```python
from build123d import *

# Parameters (mm, degrees)
BASPROSKE_W         = 4.5
BASPROSKE_H         = 48
TOOTHCUT_DEPTH      = 69.031242823
TEETHCUTS_COUNT     = 30
TEETHCUTS_ANGLE     = 348
BORSKE_R            = 5
BORE_DEPTH          = 50.0000508
BOSS_EXTRUDE2_DEPTH = 60
SKETCH6_R           = 7.7
CUT_EXTRUDE2_DEPTH  = 94.547796729


with BuildPart() as part:
    # BasProSke → Base-Revolve (revolve)
    with BuildSketch(Plane(origin=(0, 0, 0), x_dir=(1, 0, 0), z_dir=(0, 1, 0)), mode=Mode.PRIVATE) as base_revolve_sk:
        with Locations((2.25, 24)):
            Rectangle(BASPROSKE_W, BASPROSKE_H)
    revolve(base_revolve_sk.sketch.rotate(Axis((-10, 0, 0), (1, 0, 0)), 180), axis=Axis((-10, 0, 0), (1, 0, 0)))

    # TooCutSke → ToothCut (cut, through all)
    with BuildSketch(Plane(origin=(0, 0, 0), x_dir=(0, 0, -1), z_dir=(1, 0, 0))):
        with BuildLine():
            ThreePointArc((1.388358102, 41.225628713), (0, 41.249), (-1.388358102, 41.225628713))
            ThreePointArc((-1.388358102, 41.225628713), (-2.434419088, 44.674608087), (-4.146627223, 47.846050285))
            ThreePointArc((-4.146627223, 47.846050285), (0, 48.0254), (4.146627223, 47.846050285))
            ThreePointArc((4.146627223, 47.846050285), (2.434419088, 44.674608087), (1.388358102, 41.225628713))
        make_face()
    toothcut = extrude(amount=TOOTHCUT_DEPTH, mode=Mode.SUBTRACT)

    # TeethCuts: ToothCut ×30 about axis
    teethcuts_axis = Axis((-10, 0, 0), (1, 0, 0))
    for i in range(1, TEETHCUTS_COUNT):
        add(toothcut.rotate(teethcuts_axis, i * TEETHCUTS_ANGLE / (TEETHCUTS_COUNT - 1)), mode=Mode.SUBTRACT)

    # BorSke → Bore (cut, symmetric)
    with BuildSketch(Plane(origin=(0, 0, 0), x_dir=(0, 0, -1), z_dir=(1, 0, 0))):
        with Locations(Location((0, 0, 0), (0, 0, 180))):
            Circle(BORSKE_R)
    extrude(amount=BORE_DEPTH, both=True, mode=Mode.SUBTRACT)

    # Sketch5 → Boss-Extrude2 (add)
    with BuildSketch(Plane(origin=(4.5, 0, 0), x_dir=(0, 0, -1), z_dir=(1, 0, 0))):
        Polygon((22.3, 22.3), (22.3, -22.3), (-22.3, 22.3), align=None)
        Polygon((-22.3, 22.3), (-22.3, -22.3), (22.3, -22.3), align=None)
    extrude(amount=BOSS_EXTRUDE2_DEPTH)

    # Sketch6 → Cut-Extrude2 (cut, through all)
    with BuildSketch(Plane.ZY):
        Circle(SKETCH6_R)
    extrude(amount=-CUT_EXTRUDE2_DEPTH, mode=Mode.SUBTRACT)


solid = part.part
```
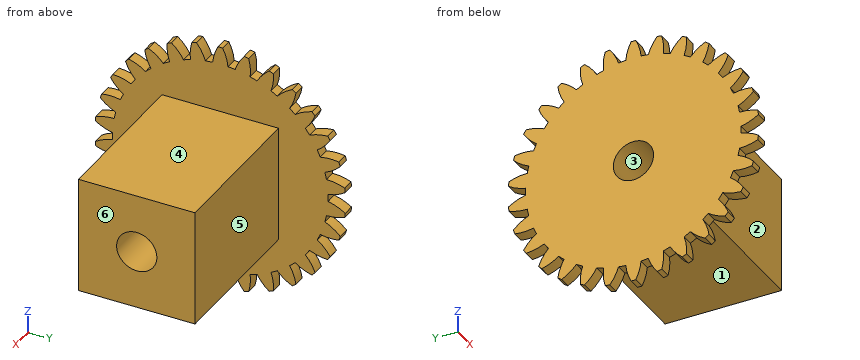
CAD build for the part. Positions are in the model's coordinates, mm. Face numbers are marked on the shaded views. A direction names the side the tool comes from. Round coordinates to 2 decimals unless told otherwise and drop trailing zeros. Loops run counter-clockwise (first coordinate to the right, second up) from the corner with the lowest first, then second, coordinate; pieces in that order, holes last. Notation, with made-up numbers: M 70.25,79 L 109.25,79 A28 ccw 109.25,113 Z; hole C -23.75,11 d5. An arc over 180 degrees is marked long. Use a Markdown table: item, result. Add a question column.
(1) Which spindle directions (+Z, -Z, +X, -X, +Y, -Y) get a long thin tool onto all of the face, cutting with end or side? Do the marked faces 4, 5 and 6. Say none if no direction does.
(2) Flat gauge pins, fed straight in: pin 1 (5 mm diameter, centred on x = 12, y = 23.5, fed in from -Z); pin 2 (10 mm diameter, centred on x = 36, z = 15.5, fed in from -Y); pin 3 (4 mm diameter, centred on x = 50, z = 23.5, fed in from +Y); pin 4 (5 mm diameter, centred on x = 54.5, y = 25, fed in from +Z). Where does each tip first touch, or does it go through?
(3) Cut at B-B (x = 59). Give the cut face in (y, z).
(4) Cut at C-C (y = 17). Give the cut face in (x, z), and give its area (3 significant figures).
(5) Drill centre lines: line 1 (Y direction, x = 49, z = 0); line 2 (Z direction, x = 45, y = 9.5); line 3 (X direction, y = -21, z = 34.5). Where is each one in solid material? Low to high.
(6) Cut at A-A (z = 0). Give the cut face in (x, y).
(7) Pull direction Z, two halves, no side cores. Call the marked faces 1, 2 and 3: +Z half, -Z half, draft (parallel to the pull), parting line (faces both ways), or undercut.
Geometry says:
| question | item | result |
|---|---|---|
| 1 | face 4 | +Z, +X, +Y, -Y |
| 1 | face 5 | +Z, -Z, +X, +Y |
| 1 | face 6 | +Z, -Z, +X, +Y, -Y |
| 2 | pin 1 | stops at z = -22.3 |
| 2 | pin 2 | stops at y = -22.3 |
| 2 | pin 3 | stops at y = 22.3 |
| 2 | pin 4 | passes through |
| 3 | outline | M -22.3,-22.3 L 22.3,-22.3 L 22.3,22.3 L -22.3,22.3 Z; hole C 0,0 d15.4 |
| 4 | outline | M 0,-42.69 L 4.5,-42.69 L 4.5,-22.3 L 64.5,-22.3 L 64.5,22.3 L 4.5,22.3 L 4.5,42.69 L 0,42.69 Z |
| 4 | area | 3,060 mm² |
| 5 | line 1 | y = -22.3 to -7.7, 7.7 to 22.3 |
| 5 | line 2 | z = -22.3 to 22.3 |
| 5 | line 3 | x = 0 to 4.5 |
| 6 | outline | M 0,-41.25 L 4.5,-41.25 L 4.5,-22.3 L 64.5,-22.3 L 64.5,-7.7 L 0,-7.7 Z; M 0,7.7 L 64.5,7.7 L 64.5,22.3 L 4.5,22.3 L 4.5,41.25 L 0,41.25 Z |
| 7 | face 1 | -Z half |
| 7 | face 2 | draft |
| 7 | face 3 | undercut |
